Input: part model. Units: mm. Frame: model coordinates. Coordinates: 2 decimals unless noted, no trailing zeros. Order: outer loops, then holes, each group sorted by start corner. A loop starts at its lowest first (then second) coordinate and runs counter-clockwise, first axis right, second up. Notation, with made-up numbers: (65, 65.25) -> (73, 65.25) arc R23 cw to (73, 97.25) -> close; hole circle Ø4 at (59, 46.25). An arc over 180 degrees is marked (long way). Write each question's results on one line, items separated by ' | '.
```python
from build123d import *

# Parameters (mm, degrees)
SKETCH1_R           = 3.96875
BOSS_EXTRUDE1_DEPTH = 7.62
FILLET1_R           = 1.27
BOSS_EXTRUDE2_START = 2.116666667
SKETCH2_R           = 5.55625
SKETCH2_R_2         = 3.96875
BOSS_EXTRUDE2_DEPTH = 2.116666667
FILLET2_R           = 1.5875
CHAMFER1_SIZE       = 0.529166836
FILLET3_R           = 0.396875


with BuildPart() as part:
    # Sketch1 → Boss-Extrude1 (new body)
    with BuildSketch(Plane.XY):
        with BuildLine():
            Line((-71.4375, 9.525), (71.4375, 9.525))
            ThreePointArc((71.4375, 9.525), (80.9625, 0), (71.4375, -9.525))
            Line((71.4375, -9.525), (-71.4375, -9.525))
            ThreePointArc((-71.4375, -9.525), (-80.9625, 0), (-71.4375, 9.525))
        make_face()
        with Locations(Location((-71.4375, 0, 0), (0, 0, 180))):
            Circle(SKETCH1_R, mode=Mode.SUBTRACT)
        with Locations(Location((71.4375, 0, 0), (0, 0, 180))):
            Circle(SKETCH1_R, mode=Mode.SUBTRACT)
    extrude(amount=BOSS_EXTRUDE1_DEPTH)

    # Fillet1
    fillet1_edges = [part.edges().sort_by_distance(p)[0] for p in [
        (80.9625, 0, 7.62),
        (0, 9.525, 7.62),
        (-80.9625, 0, 7.62),
        (0, 9.525, 0),
        (80.9625, 0, 0),
        (0, -9.525, 0),
        (-80.9625, 0, 0),
        (0, -9.525, 7.62),
    ]]
    fillet(fillet1_edges, radius=FILLET1_R)

    # Sketch2 → Boss-Extrude2 (add)
    with BuildSketch(Plane(origin=(0, 0, 0), x_dir=(-1, 0, 0), z_dir=(0, 0, -1)).offset(BOSS_EXTRUDE2_START)):
        with Locations(Location((-71.4375, 0, 0), (0, 0, 180))):
            Circle(SKETCH2_R)
        with Locations((-71.4375, 0)):
            Circle(SKETCH2_R_2, mode=Mode.SUBTRACT)
    extrude(amount=-BOSS_EXTRUDE2_DEPTH)

    # Fillet2
    fillet2_edges = [part.edges().sort_by_distance(p)[0] for p in [
        (65.88125, 0, 0),
    ]]
    fillet(fillet2_edges, radius=FILLET2_R)

    # Chamfer1
    chamfer1_edges = [part.edges().sort_by_distance(p)[0] for p in [
        (-67.46875, 0, 0),
        (-67.46875, 0, 7.62),
        (75.40625, 0, 7.62),
        (75.40625, 0, -2.116666667),
    ]]
    chamfer(chamfer1_edges, length=CHAMFER1_SIZE)

    # Fillet3
    fillet3_edges = [part.edges().sort_by_distance(p)[0] for p in [
        (65.88125, 0, -2.116666667),
    ]]
    fillet(fillet3_edges, radius=FILLET3_R)


solid = part.part
```
(1) Line query: line 1 along X through (y, z) = (0.5, 1.25); line 2 along X through (y, z) = (-3.5, 3.5); line 3 along Y through (x, z) = (26, 6.5). Output: solid intervals per line, ascending. Write a range as from..to.
Return value:
line 1: -80.95..-75.37, -67.5..67.5, 75.37..80.95 | line 2: -80.3..-73.31, -69.57..69.57, 73.31..80.3 | line 3: -9.52..9.52
(2) Pin query (flat end, axial travel): P1, Ø3, axis at x = 5, y = -2.5, coming from the -Z side; P2, Ø1, axis at x = 9.5, z = 0.5, coming from the -Y side; P3, Ø3, axis at y = 7, z = 4, coming from the +X side. Return the tip coordinate at first contact, or that it passes through.
Return value:
P1: z = 0 | P2: y = -9.5 | P3: x = 79.21
(3) Cut plane A-A, the plane y = 0. Count the separate pieces of the cut face and the enclosed holes in it, plus the area to 3 significant figures.
Return value:
separate pieces: 3 | enclosed holes: 0 | area: 1,120 mm2
(4) Mould query, pull axis Y, two halves, no side actions, for faces 1 (the face through (-80.96, -0.21, 3.77)), 2 (the face through (-75.223, -1.192, 3.764)), 3 (the face through (1, -9.525, 4)). Classes: +Y half, -Y half, draft (parallel to the pull), parting line (faces both ways), or undercut.
Return value:
face 1: parting line | face 2: undercut | face 3: -Y half
(5) Cut plane B-B, the plane x = 34.5. Return loops of the section in (y, z) (3 decimals).
Return value:
outline: (-9.525, 1.27) arc R1.27 ccw to (-8.255, 0) -> (8.255, 0) arc R1.27 ccw to (9.525, 1.27) -> (9.525, 6.35) arc R1.27 ccw to (8.255, 7.62) -> (-8.255, 7.62) arc R1.27 ccw to (-9.525, 6.35) -> close
